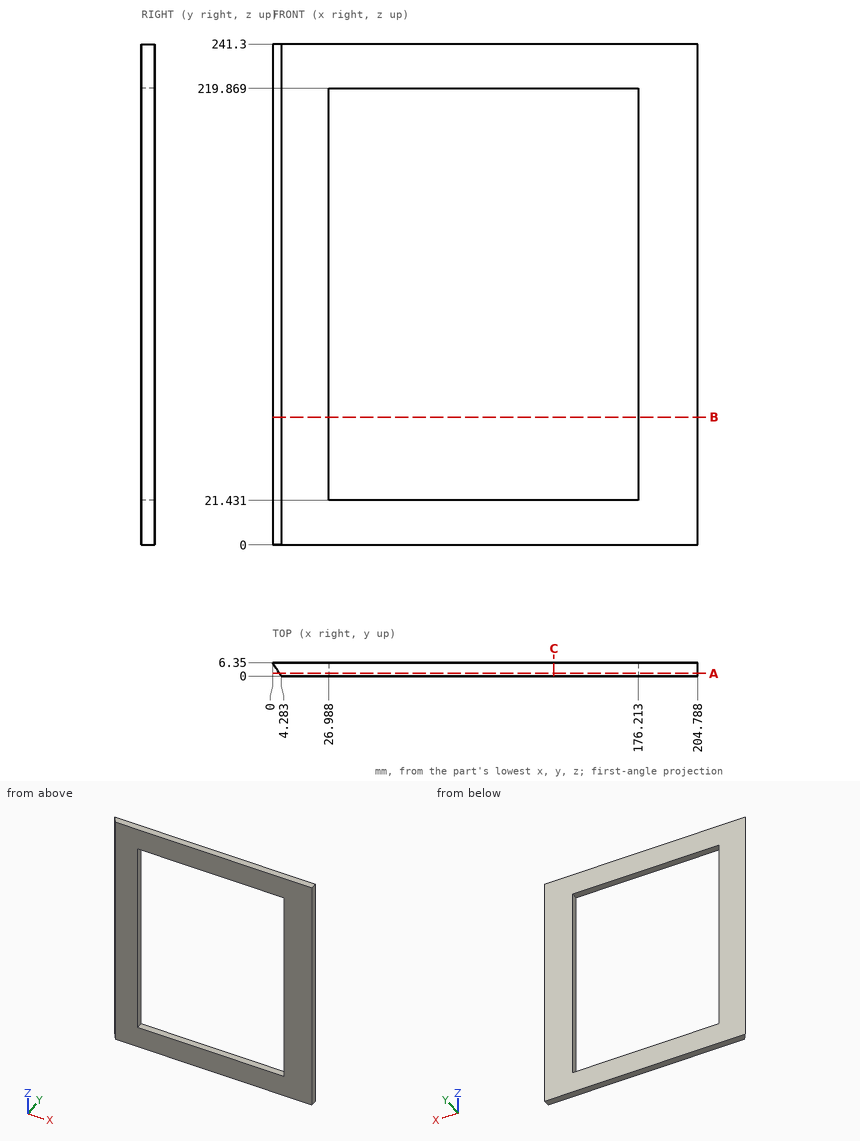
Design review of the part shown in the three views and the two pictorial views. Dimensions are in mm from the part's minimum x, y and z. Give positions to 0.01 mm unless a question says otherwise; leave off trailing zeros. Write each loop counter-clockwise with the first axis right and the second up, starting at its lowest first coordinate (ties: lowest second). Pieces come first, ordered by that corner, then holes. Notation, with made-up numbers: (52, 36.25) - (77, 36.25) arc R33 cw to (77, 66.25) - close; hole circle Ø11 at (-12.5, 77). An arc over 180 degrees is marked (long way). Return JSON: item names as keys, results as strings. Group by question number.
(1) Insertion check: pin 1 (3 mm diameter, centred on y = 2, z = 164.5, fed in from -X); pin 2 (2 mm diameter, centred on x = 87, y = 3.5, fed in from -Z); pin 3 (3 mm diameter, centred on y = 2.5, z = 200.5, fed in from -X) (1 decimal). Each pin has a flat end and moves straight along its axis. Give the tip position at first contact, or say it passes through.
(2) We need section A-A, the plane y = 1.25. Give the boundary of the cut face in (x, z), then the cut area to 3 significant figures.
(3) We need section B-B, the plane z = 61.5. Give the boundary of the cut face in (x, y).
(4) We need section C-C, the plane x = 135.5. Give the boundary of the cut face in (y, z), then the cut area to 3 significant figures.
(5) To check wall thickness, follow probe 1 along Z at (x, y) = (69, 1.5); probe 2 along X at (y, z) = (3.75, 167.5) (1 decimal); probe 3 along X at (y, z) = (5, 126). State the ranges of each line that lie inside material, in increasing order.
Reported:
{
 "1": {"pin 1": "stops at x = 1.92", "pin 2": "stops at z = 0", "pin 3": "stops at x = 1.6"},
 "2": {"outline": "(3.44, 0) - (204.79, 0) - (204.79, 241.3) - (3.44, 241.3) - close; hole (26.99, 21.43) - (176.21, 21.43) - (176.21, 219.87) - (26.99, 219.87) - close", "area": "19,000 mm2"},
 "3": {"outline": "(0, 6.35) - (4.28, 0) - (26.99, 0) - (26.99, 6.35) - close; (176.21, 0) - (204.79, 0) - (204.79, 6.35) - (176.21, 6.35) - close"},
 "4": {"outline": "(0, 0) - (6.35, 0) - (6.35, 21.43) - (0, 21.43) - close; (0, 219.87) - (6.35, 219.87) - (6.35, 241.3) - (0, 241.3) - close", "area": "272 mm2"},
 "5": {"probe 1": "z = 0 to 21.43, 219.87 to 241.3", "probe 2": "x = 1.8 to 27, 176.2 to 204.8", "probe 3": "x = 0.91 to 26.99, 176.21 to 204.79"}
}
